Study the drawing (mm; zero at the part's minimum x, y, z) and answer. A direction names the side the tool comes from. Round coordinates to 2 decimals unless told otherwise and drop trailing zeros. Write each loop counter-clockwise with the first axis right and the second up, starting at its lowest first coordinate (ties: lowest second). Pieces come first, ordered by that corner, then holes. Notation, with made-up numbers: (-27, 69.5) -> (23, 69.5) arc R15 cw to (23, 77.5) -> close; hole circle Ø6 at (52, -9.75). An arc over 180 degrees is marked (long way). Return JSON: item names as keys, results as strings.
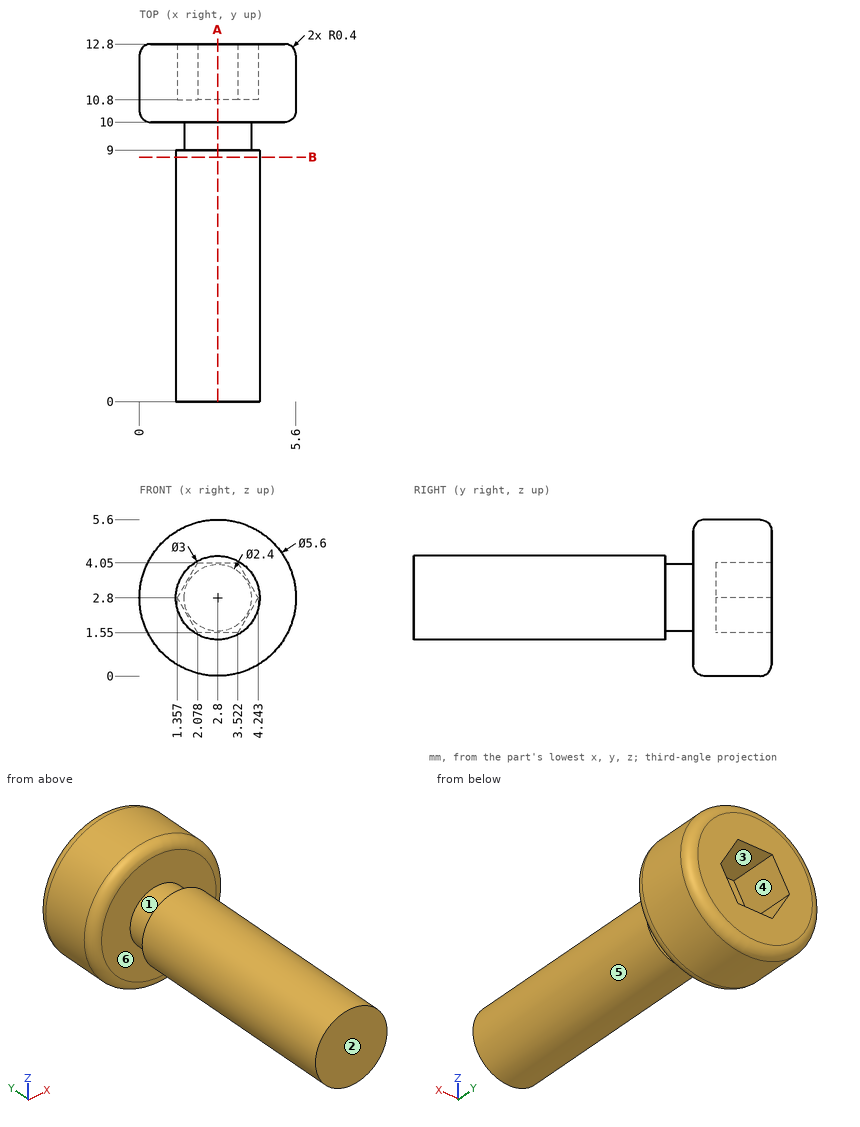
Item 1: Section B-B (y = 8.75) is taken. Give the vertices of the cut face in (x, z).
Worked answers:
{"outline": "circle Ø3 at (2.8, 2.8)"}
Item 2: A tool of negligible diameter and unlimited length cuts with its end or side. For the marked faces 1 and 2, from which of +Z, -Z, +X, -X, +Y, -Y can it reach the whole face along a straight path? Write none if from no direction.
Worked answers:
{"face 1": "none", "face 2": "+Z, -Z, +X, -X, -Y"}
Item 3: Section A-A (x = 2.8) is taken. Give the vertices of the cut face in (y, z).
Worked answers:
{"outline": "(0, 1.3) -> (9, 1.3) -> (9, 1.6) -> (10, 1.6) -> (10, 0.4) arc R0.4 ccw to (10.4, 0) -> (12.4, 0) arc R0.4 ccw to (12.8, 0.4) -> (12.8, 1.55) -> (10.8, 1.55) -> (10.8, 4.05) -> (12.8, 4.05) -> (12.8, 5.2) arc R0.4 ccw to (12.4, 5.6) -> (10.4, 5.6) arc R0.4 ccw to (10, 5.2) -> (10, 4) -> (9, 4) -> (9, 4.3) -> (0, 4.3) -> close"}
Item 4: For a pull along X with two mould halves and no side action, classify the marked faces 3, 4, 5 and 6 as released by +X, released by -X, zero draft, split by the parting line, or undercut.
Worked answers:
{"face 3": "undercut", "face 4": "undercut", "face 5": "split by the parting line", "face 6": "zero draft"}
Item 5: Straight lines are drawn through the part: L1, parallel to Y at x = 1.35, z = 4.1; L2, parallel to Z at x = 2.7, y = 2.25; L3, parallel to Y at x = 2.15, z = 2.85. For each, find the intervals that lie inside material, in ascending order. Write a range as [from, to].
Worked answers:
{"L1": "y = [10, 12.8]", "L2": "z = [1.3, 4.3]", "L3": "y = [0, 10.8]"}
Item 6: A flat-ended cylindrical pin translates along its axis: pin 1 (1 mm diameter, centred on x = 1, y = 3.5, fed in from -Z). Find the tip coordinate at first contact, or state that the pin passes through.
Worked answers:
{"pin 1": "stops at z = 2.05"}
